```python
from build123d import *

# Parameters (mm, degrees)
BOSS_EXTRUDE1_DEPTH = 3
SKETCH2_R           = 1.95
CUT_EXTRUDE1_DEPTH  = 4


with BuildPart() as part:
    # Sketch1 → Boss-Extrude1 (new body)
    with BuildSketch(Plane(origin=(0, 0, 0), x_dir=(1, 0, 0), z_dir=(0, 1, 0))):
        with BuildLine():
            Line((2, 0), (54, 0))
            ThreePointArc((54, 0), (55.414213562, -0.585786438), (56, -2))
            Line((56, -2), (56, -6))
            ThreePointArc((56, -6), (55.414213562, -7.414213562), (54, -8))
            Line((54, -8), (2, -8))
            ThreePointArc((2, -8), (0.585786438, -7.414213562), (0, -6))
            Line((0, -6), (0, -2))
            ThreePointArc((0, -2), (0.585786438, -0.585786438), (2, 0))
        make_face()
    extrude(amount=BOSS_EXTRUDE1_DEPTH)

    # Sketch2 → Cut-Extrude1 (cut, through all)
    with BuildSketch(Plane(origin=(0, 3, 0), x_dir=(1, 0, 0), z_dir=(0, 1, 0))):
        with Locations((52, -4)):
            Circle(SKETCH2_R)
        with Locations((44, -4)):
            Circle(SKETCH2_R)
        with Locations((-12, -4)):
            Circle(SKETCH2_R)
        with Locations((-4, -4)):
            Circle(SKETCH2_R)
        with Locations((4, -4)):
            Circle(SKETCH2_R)
        with Locations((12, -4)):
            Circle(SKETCH2_R)
        with Locations((20, -4)):
            Circle(SKETCH2_R)
        with Locations((28, -4)):
            Circle(SKETCH2_R)
        with Locations((36, -4)):
            Circle(SKETCH2_R)
    extrude(amount=-CUT_EXTRUDE1_DEPTH, mode=Mode.SUBTRACT)


solid = part.part
```
Could you check a few things on this model? Use its own coordinates, in mm. Round coordinates to 2 decimals unless told otherwise and drop trailing zeros. Write each loop counter-clockwise with the first axis right and the second up, starting at its lowest first coordinate (ties: lowest second). Pieces come first, ordered by that corner, then holes. Notation, with made-up numbers: M 39.5,-4.75 L 85.5,-4.75 A9 cw 85.5,3.25 Z; hole C 65.5,-22 d6. An arc over 180 degrees is marked long. Write each question's results on one line, items separated by ' | '. Start each with the question number.
1. Imagine slicing it at A-A on x = 28. List the corners of the cut face in (y, z) for me, and give its area (3 significant figures).
2. Thinking about a two-plate mould opening in X: for faces 1 (the face through (29.8, 1.52, 4.75)), 2 (the face through (0, 1, 4)), 3 (the face through (28, 0, 1)), 4 (the face through (2.453, 1.521, 5.187)), which applies, +X half, -X half, draft (parallel to the pull), parting line (faces both ways), or undercut?
3. Imagine slicing it at B-B on z = 4. Count the separate pieces of the cut face and the enclosed holes in it, and give its area (3 significant figures).
4. I need wall thicknesses on L1, parallel to Z at x = 28, y = 1; L2, parallel to Z at x = 37.5, y = 2.1; L3, parallel to X at y = 2.8, z = 1.75. Which ranges of each line are inside material? Lowest first, please. Write a range as from..to.
Result sheet:
1) outline: M 0,0 L 3,0 L 3,2.05 L 0,2.05 Z; M 0,5.95 L 3,5.95 L 3,8 L 0,8 Z | area: 12.3 mm^2
2) face 1: undercut | face 2: -X half | face 3: draft | face 4: undercut
3) separate pieces: 8 | enclosed holes: 0 | area: 86.1 mm^2
4) L1: z = 0..2.05, 5.95..8 | L2: z = 0..2.75, 5.25..8 | L3: x = 0.02..55.98
